from build123d import *

# Parameters (mm, degrees)
SKETCH1_R           = 9.525
BOSS_EXTRUDE1_DEPTH = 3.175


with BuildPart() as part:
    # Sketch1 → Boss-Extrude1 (new body, symmetric)
    with BuildSketch(Plane(origin=(0, 0, 0), x_dir=(1, 0, 0), z_dir=(0, 1, 0))):
        with BuildLine():
            Line((-25.4, 0), (-25.4, -38.1))
            ThreePointArc((-25.4, -38.1), (0, -63.5), (25.4, -38.1))
            Line((25.4, -38.1), (25.4, 0))
            Line((25.4, 0), (-25.4, 0))
        make_face()
        with Locations((0, -38.1)):
            Circle(SKETCH1_R, mode=Mode.SUBTRACT)
    extrude(amount=BOSS_EXTRUDE1_DEPTH, both=True)


solid = part.part
Check sheet for the modelled part. Datum: model origin and axes. Units: mm. Give positions to 0.01 mm unless a question says otherwise; leave off trailing zeros. Loops run counter-clockwise (first coordinate to the right, second up) from the corner with the lowest first, then second, coordinate; pieces in that order, holes last. Notation, with made-up numbers: M -16.5,17 L 40.5,17 A18 ccw 40.5,42 Z; hole C -5.5,54.5 d4. An arc over 180 degrees is marked long. Use a Markdown table: item, result. Add a question column.
Q1. Mould release check, pull along X, two halves, no side actions. Record for faces 1 (the flat face through (25.4, 0, 19)), 2 (the cylindrical face through (-1.24, -0.044, 28.656)), 3 (the cylindrical face through (-0.559, 0.044, 63.494)), 4 (the flat face through (0, 0, 0)): pulls with the +X half, pulls with the -X half, needs draft (parallel to the pull), parting line crosses it, or undercut.
Q2. Sectioned sample at A-A, the plane x = 0. Record the cut outline in (y, z) (3 decimals), then the cut area to 3 significant figures.
Q3. Sectioned sample at C-C, the plane y = 1.25. Record the cut outline in (x, z) (3 decimals), then the cut area to 3 significant figures.
Q4. Scan lines: line 1 along Z through (x, y) = (0, 1) (3 decimals); line 2 along X through (y, z) = (0.5, 38.1) (3 decimals); line 3 along X through (y, z) = (-2, 40). Record each from-to range of solid material in increasing order. Write a range as [from, to].
Q5. Sectioned sample at D-D, the plane x = -12.5. Record the cut outline in (y, z) (3 decimals), then the cut area to 3 significant figures.
Q6. Go/stop test with a flat-tipped pin: pin 1 (2 mm diameter, centred on x = 2.5, y = 1, fed in from +Z). Record where the tip stops, or that it passes through.
Q7. Sectioned sample at B-B, the plane z = 31. Record the cut outline in (x, y) (3 decimals), then the cut area to 3 significant figures.
Verdict:
| question | item | result |
|---|---|---|
| 1 | face 1 | pulls with the +X half |
| 1 | face 2 | undercut |
| 1 | face 3 | parting line crosses it |
| 1 | face 4 | needs draft |
| 2 | outline | M -3.175,0 L 3.175,0 L 3.175,28.575 L -3.175,28.575 Z; M -3.175,47.625 L 3.175,47.625 L 3.175,63.5 L -3.175,63.5 Z |
| 2 | area | 282 mm^2 |
| 3 | outline | M -25.4,0 L 25.4,0 L 25.4,38.1 A25.4 ccw -25.4,38.1 Z; hole C 0,38.1 d19.05 |
| 3 | area | 2,660 mm^2 |
| 4 | line 1 | [0, 28.575], [47.625, 63.5] |
| 4 | line 2 | [-25.4, -9.525], [9.525, 25.4] |
| 4 | line 3 | [-25.33, -9.33], [9.33, 25.33] |
| 5 | outline | M -3.175,0 L 3.175,0 L 3.175,60.211 L -3.175,60.211 Z |
| 5 | area | 382 mm^2 |
| 6 | pin 1 | z = 63.46 |
| 7 | outline | M -25.4,-3.175 L -6.349,-3.175 L -6.349,3.175 L -25.4,3.175 Z; M 6.349,-3.175 L 25.4,-3.175 L 25.4,3.175 L 6.349,3.175 Z |
| 7 | area | 242 mm^2 |
